```python
from build123d import *

# Parameters (mm, degrees)
SKETCH_1_R      = 7
EXTRUDE_1_DEPTH = 57
SKETCH_2_R      = 7.5
EXTRUDE_2_DEPTH = 10
SKETCH_3_R      = 10
EXTRUDE_3_DEPTH = 690


with BuildPart() as part:
    # 草图1 → 凸台-拉伸1 (new body)
    with BuildSketch(Plane.XY):
        with Locations(Location((0, 0, 0), (0, 0, 180))):
            Circle(SKETCH_1_R)
    extrude(amount=EXTRUDE_1_DEPTH)

    # 草图2 → 凸台-拉伸2 (add)
    with BuildSketch(Plane.XY.offset(57)):
        Circle(SKETCH_2_R)
    extrude(amount=EXTRUDE_2_DEPTH)

    # 草图3 → 凸台-拉伸3 (add)
    with BuildSketch(Plane.XY.offset(67)):
        Circle(SKETCH_3_R)
    extrude(amount=EXTRUDE_3_DEPTH)

    # 草图4 → 切除-旋转1 (revolve, cut)
    with BuildSketch(Plane(origin=(0, 0, 0), x_dir=(0, 0, -1), z_dir=(1, 0, 0)), mode=Mode.PRIVATE) as cut_revolve_1_sk:
        Polygon((-757, 0), (-757, 5), (-761.492335199, 8.145566971), (-738.304335199, 8.145566971), (-733.601489916, 0), align=None)
    revolve(cut_revolve_1_sk.sketch.rotate(Axis((0, 0, 772.39343623), (0, 0, -1)), 90), axis=Axis((0, 0, 772.39343623), (0, 0, -1)), mode=Mode.SUBTRACT)


solid = part.part
```
The listing builds one solid part. Answer for the finished solid, in the listing's coordinates (mm). A direction names the side the tool comes from. Coordinates: 2 decimals unless noted, no trailing zeros. Loops run counter-clockwise (first coordinate to the right, second up) from the corner with the lowest first, then second, coordinate; pieces in that order, holes last. Notation, with made-up numbers: M 31.5,-12.75 L 83.5,-12.75 A22 cw 83.5,26.25 Z; hole C 16.5,76 d9. An arc over 180 degrees is marked long. Answer as a JSON object with one key per item and string values. Group by question number.
Item 1: Section A-A (z = 153.5) is taken. Write down the section's boundary in (x, y), and give its area (3 significant figures).
Item 2: Each of these flat-tipped pins is pushed along its axis until it touches: P1, Ø2, axis at x = -7, z = 341, coming from the +Y side; P2, Ø2, axis at x = 7, z = 80, coming from the -Y side; P3, Ø4, axis at x = -1, y = 0, coming from the +Z side. Where does it stop, or does it pass through?
Item 3: Consider L1, parallel to Y at x = 0, z = 748.5; L2, parallel to Z at x = 8.25, y = 4; L3, parallel to Y at x = 6.75, z = 396. Determine where each line is inside the solid, lowest interval first.
Item 4: Determine the mould class of faces 4 (the face through (1.24, -0.39, 734.35)), 5 (the face through (4, 7, 67)), 6 (the face through (-2.17, -9.76, 407.17)) for opening direction Y: +Y half, -Y half, draft (parallel to the pull), parting line (faces both ways), or undercut.
Item 5: Which of the six approach directions +Z, -Z, +X, -X, +Y, -Y give full straight-line access (tool end or side, diameter ignored) to faces 1 (the face through (-7.493, 0.33, 61.93)), 2 (the face through (-1.77, 7.95, 747.52)), 3 (the face through (-3.8, -7.4, 757))?
Solved:
{
 "1": {"outline": "C 0,0 d20", "area": "314 mm2"},
 "2": {"P1": "stops at y = 8", "P2": "stops at y = -8", "P3": "stops at z = 735.33"},
 "3": {"L1": "y = -10 to -8.15, 8.15 to 10", "L2": "z = 67 to 757", "L3": "y = -7.38 to 7.38"},
 "4": {"face 4": "undercut", "face 5": "draft", "face 6": "parting line"},
 "5": {"face 1": "-Z", "face 2": "+Z", "face 3": "+Z, +X, -X, +Y, -Y"}
}
